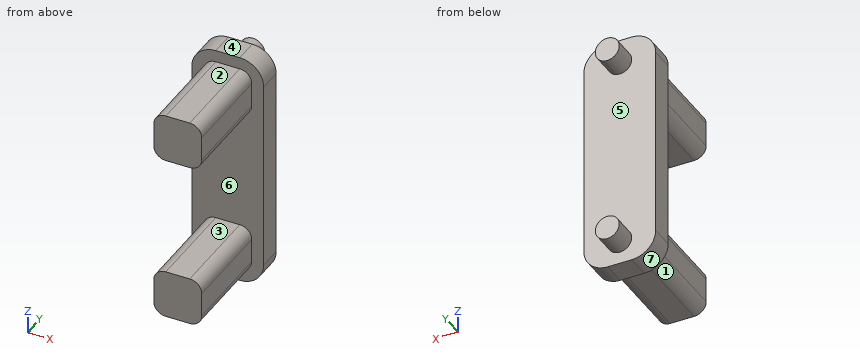
from build123d import *

# Parameters (mm, degrees)
SKETCH1_W           = 30
SKETCH1_H           = 100
BOSS_EXTRUDE1_DEPTH = 10
SKETCH2_R           = 5
BOSS_EXTRUDE2_DEPTH = 10
FILLET1_R           = 10
BOSS_EXTRUDE3_DEPTH = 40


with BuildPart() as part:
    # Sketch1 → Boss-Extrude1 (new body)
    with BuildSketch(Plane(origin=(0, 0, 0), x_dir=(1, 0, 0), z_dir=(0, 1, 0))):
        Rectangle(SKETCH1_W, SKETCH1_H)
    extrude(amount=BOSS_EXTRUDE1_DEPTH)

    # Sketch2 → Boss-Extrude2 (add)
    with BuildSketch(Plane(origin=(0, 10, 0), x_dir=(1, 0, 0), z_dir=(0, 1, 0))):
        with Locations(Location((0, 40, 0), (0, 0, 90))):
            Circle(SKETCH2_R)
        with Locations(Location((0, -40, 0), (0, 0, 90))):
            Circle(SKETCH2_R)
    extrude(amount=BOSS_EXTRUDE2_DEPTH)

    # Fillet1
    fillet1_edges = [part.edges().sort_by_distance(p)[0] for p in [
        (15, 5, 50),
        (-15, 5, 50),
        (-15, 5, -50),
        (15, 5, -50),
    ]]
    fillet(fillet1_edges, radius=FILLET1_R)

    # Sketch3 → Boss-Extrude3 (add)
    with BuildSketch(Plane.XZ):
        with BuildLine():
            Line((-10, 30), (-10, 40))
            ThreePointArc((-10, 40), (-8.535533906, 43.535533906), (-5, 45))
            Line((-5, 45), (5, 45))
            ThreePointArc((5, 45), (8.535533906, 43.535533906), (10, 40))
            Line((10, 40), (10, 30))
            ThreePointArc((10, 30), (8.535533906, 26.464466094), (5, 25))
            Line((5, 25), (-5, 25))
            ThreePointArc((-5, 25), (-8.535533906, 26.464466094), (-10, 30))
        make_face()
        with BuildLine():
            Line((5, -45), (-5, -45))
            ThreePointArc((-5, -45), (-8.535533906, -43.535533906), (-10, -40))
            Line((-10, -40), (-10, -30))
            ThreePointArc((-10, -30), (-8.535533906, -26.464466094), (-5, -25))
            Line((-5, -25), (5, -25))
            ThreePointArc((5, -25), (8.535533906, -26.464466094), (10, -30))
            Line((10, -30), (10, -40))
            ThreePointArc((10, -40), (8.535533906, -43.535533906), (5, -45))
        make_face()
    extrude(amount=BOSS_EXTRUDE3_DEPTH)


solid = part.part
Part model, mm, in its own coordinate system. Face numbers are marked on the shaded views. A direction names the side the tool comes from. Give positions to 0.01 mm unless a question says otherwise; leave off trailing zeros. Order: outer loops, then holes, each group sorted by start corner. A loop starts at its lowest first (then second) coordinate and runs counter-clockwise, first axis right, second up. Notation, with made-up numbers: (-14, 63.25) - (-3, 63.25) arc R13 cw to (-3, 87.25) - close; hole circle Ø11 at (15.5, 1.5). An arc over 180 degrees is marked (long way). One line per question, with ' | ' between items.
1. Drop flat-ended pins along their axis: P1, Ø10, axis at x = 11.5, y = -20, coming from the +Z side; P2, Ø1, axis at x = 6, y = -33, coming from the +Z side; P3, Ø6, axis at x = 7, z = -10.5, coming from the -Y side. Give the stop position or say it passes through.
Filled in:
P1: z = 44.77 | P2: z = 44.97 | P3: y = 0
2. Band-saw the part on C-C on z = -31. List the corners of the cut face in (x, y), then the cut area to 3 significant figures.
Filled in:
outline: (-15, 0) - (-10, 0) - (-10, -40) - (10, -40) - (10, 0) - (15, 0) - (15, 10) - (-15, 10) - close | area: 1,100 mm²
3. Which spindle directions (+Z, -Z, +X, -X, +Y, -Y) get a long thin tool onto all of the face, cutting with end or side? Do the marked faces 1, 2 and 3. Say none if no direction does.
Filled in:
face 1: -Z, -X, -Y | face 2: +Z, +X, -X, -Y | face 3: +X, -X, -Y
4. Drill centre lines: probe 1 along Z at (x, y) = (5.5, 5); probe 2 along Y at (x, z) = (12.5, -21); probe 3 along Z at (x, y) = (-6.5, -15.5). Where is each one in solid material? Low to high.
Filled in:
probe 1: -49.99 to 49.99 | probe 2: 0 to 10 | probe 3: -44.77 to -25.23, 25.23 to 44.77
5. Pull direction Z, two halves, no side cores. Call the marked faces 4, 5, 6 and 7: +Z half, -Z half, draft (parallel to the pull), parting line (faces both ways), or undercut.
Filled in:
face 4: +Z half | face 5: undercut | face 6: undercut | face 7: -Z half
6. Band-saw the part on D-D on y = 15.5. List the corners of the cut face in (x, z).
Filled in:
outline: circle Ø10 at (0, -40); circle Ø10 at (0, 40)
7. Band-saw the part on B-B on x = 0. List the corners of the cut face in (y, z), then the cut area to 3 significant figures.
Filled in:
outline: (-40, -45) - (0, -45) - (0, -50) - (10, -50) - (10, -45) - (20, -45) - (20, -35) - (10, -35) - (10, 35) - (20, 35) - (20, 45) - (10, 45) - (10, 50) - (0, 50) - (0, 45) - (-40, 45) - (-40, 25) - (0, 25) - (0, -25) - (-40, -25) - close | area: 2,800 mm²
8. Band-saw the part on A-A on y = -20. List the corners of the cut face in (x, z), then the cut area to 3 significant figures.
Filled in:
outline: (-10, -40) arc R5 ccw to (-5, -45) - (5, -45) arc R5 ccw to (10, -40) - (10, -30) arc R5 ccw to (5, -25) - (-5, -25) arc R5 ccw to (-10, -30) - close; (-10, 30) arc R5 ccw to (-5, 25) - (5, 25) arc R5 ccw to (10, 30) - (10, 40) arc R5 ccw to (5, 45) - (-5, 45) arc R5 ccw to (-10, 40) - close | area: 757 mm²
